```python
from build123d import *

# Parameters (mm, degrees)
EXTRUDE_1_REACH          = 233.355
SKETCH_5_W               = 270
SKETCH_5_H               = 220
SHELL_1_T                = -3
SKETCH_3_R               = 25
CUT_EXTRUDE_1_DEPTH      = 10
SKETCH_4_W               = 60
SKETCH_4_H               = 12
CUT_EXTRUDE_2_DEPTH      = 30
SKETCH_6_R               = 2.75
CUT_EXTRUDE_3_DEPTH      = 10
MIRROR_2_COPY_1_SKETCH_R = 2.75
MIRROR_2_COPY_1_DEPTH    = 10


with BuildPart() as part:
    # 草图2 → 放样2 section 0
    with BuildSketch(Plane.XY.offset(50)):
        with BuildLine():
            Line((-135, 170), (135, 170))
            Line((135, 170), (135, -50))
            Line((135, -50), (-135, -50))
            Line((-135, -50), (-135, 170))
        make_face()
    # 草图1 → 放样2 section 1
    with BuildSketch(Plane.XY):
        with BuildLine():
            Line((-30, 30), (30, 30))
            Line((30, 30), (30, -30))
            Line((30, -30), (-30, -30))
            Line((-30, -30), (-30, 30))
        make_face()
    loft()

    # 草图5 → 凸台-拉伸1 (add, up to next)
    with BuildSketch(Plane.XY.offset(80), mode=Mode.PRIVATE) as extrude_1_sk1:
        with Locations((0, 60)):
            Rectangle(SKETCH_5_W, SKETCH_5_H)
    extrude_1_tool1 = extrude(extrude_1_sk1.sketch, amount=-EXTRUDE_1_REACH, mode=Mode.PRIVATE) - part.part
    add(extrude_1_tool1.solids().sort_by_distance((0, 60, 80))[0])

    # 抽壳1
    shell_1_openings = [part.faces().sort_by_distance(p)[0] for p in [
        (0, 60, 80),
    ]]
    offset(amount=SHELL_1_T, openings=shell_1_openings)

    # 草图3 → 切除-拉伸1 (cut)
    with BuildSketch(Plane.XY.offset(3)):
        Circle(SKETCH_3_R)
    extrude(amount=-CUT_EXTRUDE_1_DEPTH, mode=Mode.SUBTRACT)

    # 草图4 → 切除-拉伸2 (cut)
    with BuildSketch(Plane(origin=(0, 0, 0), x_dir=(-1, 0, 0), z_dir=(0, 0, -1))):
        with Locations((0, 36)):
            Rectangle(SKETCH_4_W, SKETCH_4_H)
    extrude(amount=-CUT_EXTRUDE_2_DEPTH, mode=Mode.SUBTRACT)

    # 草图6 → 切除-拉伸3 (cut)
    with BuildSketch(Plane.XZ.offset(50)):
        with Locations(Location((65.65, 65, 0), (0, 0, 270))):
            Circle(SKETCH_6_R)
        with Locations(Location((76.65, 65, 0), (0, 0, 270))):
            Circle(SKETCH_6_R)
        with Locations(Location((87.65, 65, 0), (0, 0, 270))):
            Circle(SKETCH_6_R)
        with Locations(Location((109.65, 65, 0), (0, 0, 270))):
            Circle(SKETCH_6_R)
    cut_extrude_3 = extrude(amount=-CUT_EXTRUDE_3_DEPTH, mode=Mode.SUBTRACT)

    # 镜向1: 切除-拉伸3 across plane
    add(cut_extrude_3.mirror(Plane(origin=(0, 60, 0), x_dir=(0, 0, 1), z_dir=(0, -1, 0))), mode=Mode.SUBTRACT)

    # 镜向2: 切除-拉伸3 across plane
    add(cut_extrude_3.mirror(Plane(origin=(0, 0, 0), x_dir=(0, 0, 1), z_dir=(1, 0, 0))), mode=Mode.SUBTRACT)

    # 镜向2 copy 1 sketch → 镜向2 copy 1 (cut)
    with BuildSketch(Plane(origin=(0, 170, 0), x_dir=(-1, 0, 0), z_dir=(0, 1, 0))):
        with Locations(Location((65.65, 65, 0), (0, 0, 270))):
            Circle(MIRROR_2_COPY_1_SKETCH_R)
        with Locations(Location((76.65, 65, 0), (0, 0, 270))):
            Circle(MIRROR_2_COPY_1_SKETCH_R)
        with Locations(Location((87.65, 65, 0), (0, 0, 270))):
            Circle(MIRROR_2_COPY_1_SKETCH_R)
        with Locations(Location((109.65, 65, 0), (0, 0, 270))):
            Circle(MIRROR_2_COPY_1_SKETCH_R)
    extrude(amount=-MIRROR_2_COPY_1_DEPTH, mode=Mode.SUBTRACT)


solid = part.part
```
Check sheet for the modelled part. Datum: model origin and axes. Units: mm. A direction names the side the tool comes from. Coordinates: 2 decimals unless noted, no trailing zeros. Order: outer loops, then holes, each group sorted by start corner. A loop starts at its lowest first (then second) coordinate and runs counter-clockwise, first axis right, second up. Notation, with made-up numbers: (28, 37.25) -> (57, 37.25) arc R15 cw to (57, 62.25) -> close; hole circle Ø9 at (81.5, 89). An arc over 180 degrees is marked (long way). Write item = value, one per line. Start each with the question number.
1) Mould release check, pull along X, two halves, no side actions. Record for faces 1 (the flat face through (-2, -50, 65)), 2 (the flat face through (135, 58, 65)), 3 (the flat face through (-132, 59, 66)): +X half, -X half, draft (parallel to the pull), parting line (faces both ways), or undercut.
2) Material ranges on L1, parallel to X at y = 119, z = 76.5; L2, parallel to Y at x = 3, z = 60.5; L3, parallel to X at y = 108.5, z = 37.5, recorded low to high.
3) Go/stop test with flat-tipped pins: P1, Ø3.5, axis at x = -109.65, z = 65, coming from the -Y side; P2, Ø8, axis at y = 34.5, z = 4.5, coming from the -X side; P3, Ø8, axis at y = 24.5, z = 31, coming from the -X side; P4, Ø12, axis at x = -71.5, y = 20, coming from the -Z side. Record where each tip stops, or that it passes through.
4) Cross-section at A-A (z = 74.5). Enter the section's corners in (x, y).
5) Access from +Z, -Z, +X, -X, +Y, -Y to the whole of each face (thin tool, end or side, straight path). Record for faces 4 (the cylindrical face through (76.771, 168.521, 67.747)), 5 (the flat face through (-2, 167, 66)), 6 (the flat face through (-30, 36, 4)), 7 (the flat face through (-2, 170, 65)).
6) Cross-section at B-B (x = 0). State how many separate pieces and enclosed holes the cut face has, then the cut area to 3 significant figures.
Ans:
q1.face_1 = draft
q1.face_2 = +X half
q1.face_3 = undercut
q2.L1 = -135 to -132, 132 to 135
q2.L2 = -50 to -47, 167 to 170
q2.L3 = -108.75 to -101.77, 101.77 to 108.75
q3.P1 = through
q3.P2 = -47.85
q3.P3 = -103.5
q3.P4 = 16.9
q4.outline = (-135, -50) -> (135, -50) -> (135, 170) -> (-135, 170) -> close; hole (-132, -47) -> (132, -47) -> (132, 167) -> (-132, 167) -> close
q5.face_4 = +Y, -Y
q5.face_5 = +Z
q5.face_6 = +Z, -Z
q5.face_7 = +Z, -Z, +X, -X, +Y
q6.separate_pieces = 3
q6.enclosed_holes = 0
q6.area = 764 mm²
